Autodesk Inventor part; units mm, degrees
ref_plane "YZ Plane" through (0, 0, 0) normal (1, 0, 0) x (0, 1, 0)
ref_plane "XZ Plane" through (0, 0, 0) normal (0, 1, 0) x (-1, 0, 0)
ref_plane "XY Plane" through (0, 0, 0) normal (0, 0, 1) x (1, 0, 0)
sketch "Sketch1" plane through (0, 0, 0) normal (0, 0, 1) x (1, 0, 0)
  line L0 (0, 0) -> (140, 0)
  line L1 (140, 0) -> (140, 140)
  line L2 (140, 140) -> (0, 140)
  line L3 (0, 140) -> (0, 0)
  dimension "d0" = 140
  dimension "d1" = 140
extrude "Extrusion1" add sketch "Sketch1" along normal blind 3
fillet "Fillet1" radius 5 4 edges at (140, 140, 1.5) (140, 0, 1.5) (0, 140, 1.5) (0, 0, 1.5)
sketch "Sketch2" plane through (0, 0, 3) normal (0, 0, 1) x (1, 0, 0)
  circle A0 centre (20, 110) radius 2.5
  line L0 (135, 140) -> (5, 140)
  line L1 (0, 135) -> (0, 5)
  circle A1 centre (69, 110) radius 2.5
  circle A2 centre (20, 52) radius 2.5
  circle A3 centre (69, 52) radius 2.5
  point P0 (0, 0)
  dimension "d5" = 5
  dimension "d6" = 30
  dimension "d7" = 20
  dimension "d8" = 5
  dimension "d9" = 30
  dimension "d10" = 69
  dimension "d11" = 5
  dimension "d12" = 20
  dimension "d13" = 88
  dimension "d14" = 5
  dimension "d15" = 88
  dimension "d16" = 69
extrude "Extrusion2" add sketch "Sketch2" along normal blind 3
sketch "Sketch3" plane through (20, 110, 6) normal (0, 0, 1) x (1, 0, 0)
  circle A0 centre (0, 0) radius 1.35
  circle A1 centre (49, 0) radius 2.5
  circle A2 centre (49, 0) radius 1.35
  circle A3 centre (0, -58) radius 2.5
  circle A4 centre (0, -58) radius 1.35
  circle A5 centre (49, -58) radius 2.5
  circle A6 centre (49, -58) radius 1.35
  point P0 (-20, -110)
  dimension "d19" = 2.7
  dimension "d20" = 2.7
extrude "Extrusion3" add sketch "Sketch3" along normal blind 2 contours A0 | A2 | A4 | A6
sketch "Sketch4" plane through (0, 0, 3) normal (0, 0, 1) x (1, 0, 0)
  line L0 (135, 140) -> (5, 140)
  line L1 (0, 135) -> (0, 5)
  line L2 (140, 5) -> (140, 135)
  line L3 (5, 0) -> (135, 0)
  point P0 (0, 0)
  point P1 (6, 134)
  point P2 (134, 134)
  point P3 (6, 6)
  point P4 (134, 6)
  dimension "d30" = 6
  dimension "d31" = 6
  dimension "d32" = 6
  dimension "d33" = 6
  dimension "d34" = 6
  dimension "d35" = 6
  dimension "d36" = 6
  dimension "d37" = 6
hole "Hole2" at (134, 134, 3) at (6, 6, 3) at (134, 6, 3) at (6, 134, 3) direction (0, 0, -1) diameter 4 depth 15
sketch "Sketch5" plane through (0, 0, 3) normal (0, 0, 1) x (1, 0, 0)
  line L0 (20, 130) -> (120, 130)
  line L1 (120, 130) -> (120, 125)
  line L2 (120, 125) -> (20, 125)
  line L3 (20, 125) -> (20, 130)
  line L4 (135, 140) -> (5, 140)
  line L5 (140, 5) -> (140, 135)
  line L6 (20, 15) -> (120, 15)
  line L7 (120, 15) -> (120, 10)
  line L8 (120, 10) -> (20, 10)
  line L9 (20, 10) -> (20, 15)
  line L10 (5, 0) -> (135, 0)
  line L11 (10, 120) -> (15, 120)
  line L12 (15, 120) -> (15, 20)
  line L13 (15, 20) -> (10, 20)
  line L14 (10, 20) -> (10, 120)
  line L15 (0, 135) -> (0, 5)
  line L16 (125, 120) -> (130, 120)
  line L17 (130, 120) -> (130, 20)
  line L18 (130, 20) -> (125, 20)
  line L19 (125, 20) -> (125, 120)
  point P0 (0, 0)
  dimension "d45" = 10
  dimension "d46" = 5
  dimension "d47" = 20
  dimension "d48" = 100
  dimension "d49" = 100
  dimension "d50" = 5
  dimension "d51" = 20
  dimension "d52" = 10
  dimension "d53" = 5
  dimension "d54" = 100
  dimension "d55" = 20
  dimension "d56" = 10
  dimension "d57" = 5
  dimension "d58" = 100
  dimension "d59" = 10
  dimension "d60" = 20
extrude "Extrusion4" cut sketch "Sketch5" against normal blind 10
sketch "Sketch6" plane through (0, 0, 3) normal (0, 0, 1) x (1, 0, 0)
  circle A0 centre (100, 85) radius 2.5
  line L0 (140, 5) -> (140, 135)
  line L1 (135, 140) -> (5, 140)
  point P0 (0, 0)
  dimension "d63" = 5
  dimension "d66" = 40
  dimension "d67" = 55
extrude "Extrusion5" add sketch "Sketch6" along normal blind 3
sketch "Sketch7" plane through (100, 85, 6) normal (0, 0, 1) x (1, 0, 0)
  circle A0 centre (0, 0) radius 1.75
  point P0 (-100, -85)
  dimension "d68" = 3.5
extrude "Extrusion6" add sketch "Sketch7" along normal blind 4
sketch "Sketch8" plane through (0, 0, 3) normal (0, 0, 1) x (1, 0, 0)
  line L0 (90, 75) -> (110, 75)
  line L1 (110, 75) -> (110, 70)
  line L2 (110, 70) -> (90, 70)
  line L3 (90, 70) -> (90, 75)
  line L4 (140, 5) -> (140, 135)
  line L5 (5, 0) -> (135, 0)
  point P0 (0, 0)
  dimension "d71" = 20
  dimension "d72" = 30
  dimension "d73" = 5
  dimension "d74" = 70
extrude "Extrusion7" add sketch "Sketch8" along normal blind 6
sketch "Sketch9" plane through (0, 0, 9) normal (0, 0, 1) x (1, 0, 0)
  line L0 (90, 75) -> (110, 75)
  line L1 (110, 70) -> (90, 70)
  line L2 (92.5, 75) -> (107.5, 75)
  line L3 (107.5, 75) -> (107.5, 70)
  line L4 (107.5, 70) -> (92.5, 70)
  line L5 (92.5, 70) -> (92.5, 75)
  line L6 (110, 70) -> (110, 75)
  line L7 (90, 75) -> (90, 70)
  point P0 (0, 0)
  dimension "d77" = 2.5
  dimension "d78" = 2.5
extrude "Extrusion8" cut sketch "Sketch9" against normal blind 3 contours L0 L3 L1 L5
chamfer "Chamfer1" distance 2 angle 45 4 edges at (6, 8, 0) (134, 8, 0) (6, 136, 0) (134, 136, 0)
properties part number "Led deksel"
Design review of the part built by this model. Coordinates are the model's own, in mm. A direction names the side the tool comes from. Coordinates: 2 decimals unless noted, no trailing zeros. Write each loop counter-clockwise with the first axis right and the second up, starting at its lowest first coordinate (ties: lowest second). Pieces come first, ordered by that corner, then holes. Notation, with made-up numbers: M 1,-26 L 20,-26 A19 ccw 20,-14 Z; hole C 70,28.5 d11. An arc over 180 degrees is marked long. Answer as a JSON object with one key per item and string values.
Item 1: Draft analysis for pull direction X (two halves, no side actions). For faces 1 (the flat face through (110, 73, 6)), 2 (the flat face through (13, 20, 2)), 3 (the flat face through (69, 0, 1)), state which applies: pulls with the +X half, pulls with the -X half, needs draft (parallel to the pull), parting line crosses it, or undercut.
Outcome:
{"face 1": "pulls with the +X half", "face 2": "undercut", "face 3": "needs draft"}
Item 2: Add section D-D, the plane x = 100. Give the boundary of the cut face in (y, z).
Outcome:
{"outline": "M 0,0 L 10,0 L 10,3 L 0,3 Z; M 15,0 L 125,0 L 125,3 L 87.5,3 L 87.5,6 L 86.75,6 L 86.75,10 L 83.25,10 L 83.25,6 L 82.5,6 L 82.5,3 L 75,3 L 75,6 L 70,6 L 70,3 L 15,3 Z; M 130,0 L 140,0 L 140,3 L 130,3 Z"}
Item 3: Add section C-C, the plane y = 85. Give the boundary of the cut face in (x, z), and give its area (3 significant figures).
Outcome:
{"outline": "M 0,0 L 10,0 L 10,3 L 0,3 Z; M 15,0 L 125,0 L 125,3 L 102.5,3 L 102.5,6 L 101.75,6 L 101.75,10 L 98.25,10 L 98.25,6 L 97.5,6 L 97.5,3 L 15,3 Z; M 130,0 L 140,0 L 140,3 L 130,3 Z", "area": "419 mm²"}
Item 4: Add section A-A, the plane x = 80.5. Give the boundary of the cut face in (y, z).
Outcome:
{"outline": "M 0,0 L 10,0 L 10,3 L 0,3 Z; M 15,0 L 125,0 L 125,3 L 15,3 Z; M 130,0 L 140,0 L 140,3 L 130,3 Z"}
Item 5: Insertion check: pin 1 Ø3 at (x, z) = (106.5, 9) entering from -Y; pin 2 Ø2.5 at (y, z) = (72, 5.5) entering from -X; pin 3 Ø2.5 at (x, y) = (19, 51.5) entering from +Z; pin 4 Ø2 at (x, z) = (122.5, 5.5) entering from +Y. Each pin has a flat end and moves straight along its axis. Give the tip position at first contact, or say it passes through.
Outcome:
{"pin 1": "y = 70", "pin 2": "x = 90", "pin 3": "z = 8", "pin 4": "through"}
Item 6: Machinability: for faces 4 (the flat face through (70.1, 50.9, 6)), 5 (the flat face through (107.5, 73, 8)), 6 (the flat face through (71, 10, 2)), which of the approach directions +Z, -Z, +X, -X, +Y, -Y give a long, thin tool a straight path to every point of the face, cutting with its end or side? Answer none if there is none.
Outcome:
{"face 4": "+Z", "face 5": "+Z, +Y, -Y", "face 6": "+Z, -Z"}
Item 7: Wall thickness on probe 1 along X at (y, z) = (69.5, 2.75); probe 2 along Y at (x, z) = (134, 2.65): over which ranges is each line inside the solid? List them lowest first.
Outcome:
{"probe 1": "0 to 10, 15 to 125, 130 to 140", "probe 2": "0 to 4, 8 to 132, 136 to 140"}
